Check sheet for the modelled part. Datum: model origin and axes. Units: mm. A direction names the side the tool comes from. Coordinates: 2 decimals unless noted, no trailing zeros. Loops run counter-clockwise (first coordinate to the right, second up) from the corner with the lowest first, then second, coordinate; pieces in that order, holes last. Notation, with made-up numbers: (64, 56.5) - (100, 56.5) arc R12 ccw to (100, 78.5) - close; hole circle Ø3 at (-18, -8.75). An arc over 180 degrees is marked (long way). Use a Markdown table: item, result. Add a question column.
1) Draft check along Y on faces 3 (the flat face through (-21, -8.169, 20)), 4 (the cylindrical face through (-22.33, 6.38, 1.97)), 5 (the flat face through (-29, 12, 4)). Enter one of: pulls with the +Y half, pulls with the -Y half, needs draft (parallel to the pull), parting line crosses it, or undercut.
2) Sectioned sample at C-C, the plane y = 20. Enter the section's corners in (x, z), then the cut area to 3 significant figures.
3) Sectioned sample at A-A, the plane z = 19. Enter the section's corners in (x, y).
4) Go/stop test with flat-tipped pins: P1, Ø18, axis at x = -17.5, y = 30, coming from the +Z side; P2, Ø4, axis at x = -20.9, y = 6.83, coming from the -Z side; P3, Ø1, axis at x = -32.5, z = 8, coming from the +Y side. Record where each tip stops, or that it passes through.
5) Sectioned sample at B-B, the plane x = -15. Enter the section's corners in (y, z).
6) Tool access check on faces 1 (the flat face through (-2.9, -5, 13)), 2 (the flat face through (-21, -4.169, 24)). Record the directions out of +Z, -Z, +X, -X, +Y, -Y that give a thin tool (end or side, any length) a straight path to the whole face; none if there is none.
7) Sectioned sample at D-D, the plane z = 10.5. Enter the section's corners in (x, y).
8) Thickness scan on line 1 (X direction, y = -6, z = 19); line 2 (Z direction, x = -33.5, y = 8); line 3 (Y direction, x = -19.5, z = 17). Record the ranges inside material, lowest first.
from build123d import *

# Parameters (mm, degrees)
BOSS_EXTRUDE1_DEPTH = 4
SKETCH3_W           = 36
SKETCH3_H           = 4
BOSS_EXTRUDE2_DEPTH = 40
SKETCH4_R           = 11
SKETCH4_R_2         = 1.5
CUT_EXTRUDE1_DEPTH  = 22
SKETCH5_R           = 1.5
CUT_EXTRUDE2_DEPTH  = 10
BOSS_EXTRUDE4_DEPTH = 36


with BuildPart() as part:
    # Sketch1 → Boss-Extrude1 (new body)
    with BuildSketch(Plane.XY):
        with BuildLine():
            Line((-38.900365485, 21.830923248), (-38.900365485, -8.169076752))
            Line((-38.900365485, -8.169076752), (-2.900365485, -8.169076752))
            Line((-2.900365485, -8.169076752), (-2.900365485, 21.830923248))
            ThreePointArc((-2.900365485, 21.830923248), (-20.900365485, 39.830923248), (-38.900365485, 21.830923248))
        make_face()
    extrude(amount=BOSS_EXTRUDE1_DEPTH)

    # Sketch3 → Boss-Extrude2 (add)
    with BuildSketch(Plane.XY):
        with Locations((-20.900365485, -6.169076752)):
            Rectangle(SKETCH3_W, SKETCH3_H)
    extrude(amount=BOSS_EXTRUDE2_DEPTH)

    # Sketch4 → Cut-Extrude1 (cut)
    with BuildSketch(Plane.XY):
        with Locations(Location((-20.900365485, 21.830923248, 0), (0, 0, 180))):
            Circle(SKETCH4_R)
        with Locations(Location((-20.900365485, 6.830923248, 0), (0, 0, 180))):
            Circle(SKETCH4_R_2)
        with Locations(Location((-33.890746542, 29.330923248, 0), (0, 0, 180))):
            Circle(SKETCH4_R_2)
        with Locations(Location((-7.909984429, 29.330923248, 0), (0, 0, 180))):
            Circle(SKETCH4_R_2)
    extrude(amount=CUT_EXTRUDE1_DEPTH, mode=Mode.SUBTRACT)

    # Sketch5 → Cut-Extrude2 (cut)
    with BuildSketch(Plane(origin=(0, 0, 0), x_dir=(1, 0, 0), z_dir=(0, 1, 0))):
        with Locations(Location((-28.900365485, -19, 0), (0, 0, 270))):
            Circle(SKETCH5_R)
        with Locations(Location((-12.900365485, -19, 0), (0, 0, 270))):
            Circle(SKETCH5_R)
        with Locations(Location((-20.900365485, -34.884, 0), (0, 0, 270))):
            Circle(SKETCH5_R)
    extrude(amount=-CUT_EXTRUDE2_DEPTH, mode=Mode.SUBTRACT)

    # Sketch7 → Boss-Extrude4 (add)
    with BuildSketch(Plane(origin=(-2.900365485, 0, 0), x_dir=(0, 0, -1), z_dir=(1, 0, 0))):
        Polygon((-4, 0.364546523), (-7.977975303, -4.169076752), (-4, -4.169076752), align=None)
    extrude(amount=-BOSS_EXTRUDE4_DEPTH)


solid = part.part
Solved:
| question | item | result |
|---|---|---|
| 1 | face 3 | pulls with the -Y half |
| 1 | face 4 | undercut |
| 1 | face 5 | needs draft |
| 2 | outline | (-38.9, 0) - (-31.75, 0) - (-31.75, 4) - (-38.9, 4) - close; (-10.05, 0) - (-2.9, 0) - (-2.9, 4) - (-10.05, 4) - close |
| 2 | area | 57.2 mm2 |
| 3 | outline | (-38.9, -8.17) - (-30.4, -8.17) - (-30.4, -4.17) - (-38.9, -4.17) - close; (-27.4, -8.17) - (-14.4, -8.17) - (-14.4, -4.17) - (-27.4, -4.17) - close; (-11.4, -8.17) - (-2.9, -8.17) - (-2.9, -4.17) - (-11.4, -4.17) - close |
| 4 | P1 | stops at z = 4 |
| 4 | P2 | stops at z = 0 |
| 4 | P3 | stops at y = -3.62 |
| 5 | outline | (-8.17, 0) - (12.55, 0) - (12.55, 4) - (0.36, 4) - (-4.17, 7.98) - (-4.17, 40) - (-8.17, 40) - close; (31.11, 0) - (38.84, 0) - (38.84, 4) - (31.11, 4) - close |
| 6 | face 1 | +Z, -Z, +X, +Y, -Y |
| 6 | face 2 | +Z, +X, -X, +Y |
| 7 | outline | (-38.9, -8.17) - (-2.9, -8.17) - (-2.9, -4.17) - (-38.9, -4.17) - close |
| 8 | line 1 | x = -38.9 to -30.4, -27.4 to -14.4, -11.4 to -2.9 |
| 8 | line 2 | z = 0 to 4 |
| 8 | line 3 | y = -8.17 to -4.17 |
